```python
from build123d import *

# Parameters (mm, degrees)
F0_R     = 12.7
F1_DEPTH = 38.1
F3_DEPTH = 234.95
F5_DEPTH = 31.75
F6_SIZE  = 19.05


with BuildPart() as f1:
    # F0 (on Right) → F1 (new body)
    with BuildSketch(Plane.YZ):
        Polygon((0, 38.1), (0, 0), (50.8, 0), (50.8, 16.51), (31.75, 16.51), (31.75, 29.21), (50.8, 29.21), (50.8, 38.1), align=None)
        with BuildLine():
            Line((0, 50.8), (0, 38.1))
            Line((0, 38.1), (50.8, 38.1))
            Line((50.8, 38.1), (76.2, 38.1))
            Line((76.2, 38.1), (127, 38.1))
            Line((127, 38.1), (127, 50.8))
            Line((127, 50.8), (111.125, 50.8))
            Line((111.125, 50.8), (84.5934256055, 90.3501730104))
            ThreePointArc((84.5934256055, 90.3501730104), (63.5, 101.6), (42.4065743945, 90.3501730104))
            Line((42.4065743945, 90.3501730104), (15.875, 50.8))
            Line((15.875, 50.8), (0, 50.8))
        make_face()
        with Locations((63.5, 76.2)):
            Circle(F0_R, mode=Mode.SUBTRACT)
        Polygon((127, 38.1), (76.2, 38.1), (76.2, 29.21), (95.25, 29.21), (95.25, 16.51), (76.2, 16.51), (76.2, 0), (127, 0), align=None)
    extrude(amount=-F1_DEPTH)

    # F2 (on face) → F3 (join)
    with BuildSketch(Plane(origin=(-38.1, 0, 0), x_dir=(0, -1, 0), z_dir=(-1, 0, 0))):
        Polygon((0, 38.1), (-50.8, 38.1), (-50.8, 29.21), (-31.75, 29.21), (-31.75, 16.51), (-50.8, 16.51), (-50.8, 0), (0, 0), align=None)
        Polygon((-76.2, 38.1), (-127, 38.1), (-127, 0), (-76.2, 0), (-76.2, 16.51), (-95.25, 16.51), (-95.25, 29.21), (-76.2, 29.21), align=None)
    extrude(amount=F3_DEPTH)

    # F4 (on face) → F5 (join)
    with BuildSketch(Plane(origin=(-273.05, 0, 0), x_dir=(0, -1, 0), z_dir=(-1, 0, 0))):
        Polygon((-76.2, 16.51), (-76.2, 0), (0, 0), (0, 101.6), (-127, 101.6), (-127, 38.1), (-76.2, 38.1), (-76.2, 29.21), (-95.25, 29.21), (-95.25, 16.51), align=None)
        Polygon((-127, 38.1), (-127, 0), (-76.2, 0), (-76.2, 16.51), (-95.25, 16.51), (-95.25, 29.21), (-76.2, 29.21), (-76.2, 38.1), align=None)
    extrude(amount=F5_DEPTH)

    # F6
    f6_edges = [f1.edges().sort_by_distance(p)[0] for p in [
        (-304.8, 63.5, 101.6),
    ]]
    chamfer(f6_edges, length=F6_SIZE)


solid = f1.part
```
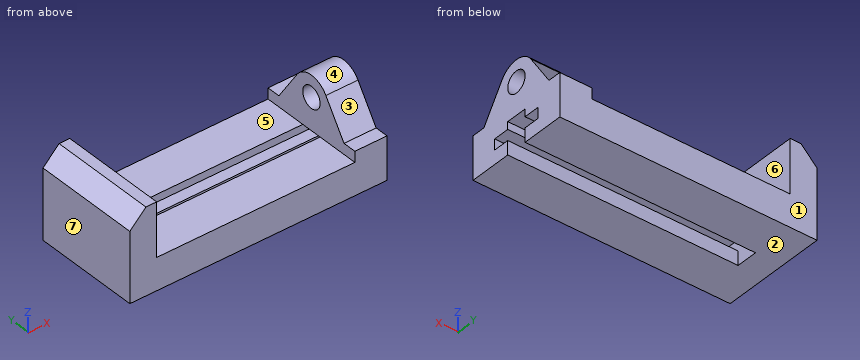
Check sheet for the modelled part. Datum: model origin and axes. Units: mm. Face numbers are marked on the shaded views. A direction names the side the tool comes from. Give positions to 0.01 mm unless a question says otherwise; leave off trailing zeros. Write each loop counter-clockwise with the first axis right and the second up, starting at its lowest first coordinate (ties: lowest second). Pieces come first, ordered by that corner, then holes. Notation, with made-up numbers: (5, -38) - (16, -38) arc R19 ccw to (16, -23) - close; hole circle Ø11 at (63.25, 28). An arc over 180 degrees is marked (long way). Answer as a JSON object with one key per item and string values. Group by question number.
1) Sectioned sample at C-C (z = 59). Record the cut outline in (x, y), then the cut area to 3 significant figures.
2) Thickness scan on probe 1 along Y at (x, z) = (-191, 6.5); probe 2 along X at (y, z) = (47.5, 80); probe 3 along Z at (x, y) = (-246.5, 94). Record the ranges inside material, lowest first. Write a range as from..to.
3) Sectioned sample at D-D (z = 76.2). Record the cut outline in (x, y), then the cut area to 3 significant figures.
4) Access from +Z, -Z, +X, -X, +Y, -Y to the whole of each face (thin tool, end or side, straight path). Record for the marked faces 4, 5, 6 and 7.
5) Sectioned sample at A-A (x = -147). Record the cut outline in (y, z).
6) Depth check by flat-ended pin: P1, Ø8, axis at x = -27, y = 117.5, coming from the +Z side. Enter the tip coordinate at first touch or a pass-through.
7) Sectioned sample at B-B (y = 63.5). Record the cut outline in (x, z).
8) Release check for a two-part mould opening along Z. For the marked faces 1, 2 and 3 record: pulls with the +Z half, pulls with the -Z half, needs draft (parallel to the pull), parting line crosses it, or undercut.
Geometry results:
{
 "1": {"outline": "(-304.8, 0) - (-273.05, 0) - (-273.05, 127) - (-304.8, 127) - close; (-38.1, 21.38) - (0, 21.38) - (0, 105.62) - (-38.1, 105.62) - close", "area": "7,240 mm^2"},
 "2": {"probe 1": "y = 0..50.8, 76.2..127", "probe 2": "x = -304.8..-273.05, -38.1..0", "probe 3": "z = 0..16.51, 29.21..38.1"},
 "3": {"outline": "(-304.8, 0) - (-273.05, 0) - (-273.05, 127) - (-304.8, 127) - close; (-38.1, 32.91) - (0, 32.91) - (0, 50.8) - (-38.1, 50.8) - close; (-38.1, 76.2) - (0, 76.2) - (0, 94.09) - (-38.1, 94.09) - close", "area": "5,400 mm^2"},
 "4": {"face 4": "+Z, +X", "face 5": "+Z, +Y, -Y", "face 6": "none", "face 7": "+Z, -Z, -X, +Y, -Y"},
 "5": {"outline": "(0, 0) - (50.8, 0) - (50.8, 16.51) - (31.75, 16.51) - (31.75, 29.21) - (50.8, 29.21) - (50.8, 38.1) - (0, 38.1) - close; (76.2, 0) - (127, 0) - (127, 38.1) - (76.2, 38.1) - (76.2, 29.21) - (95.25, 29.21) - (95.25, 16.51) - (76.2, 16.51) - close"},
 "6": {"P1": "stops at z = 50.8"},
 "7": {"outline": "(-304.8, 0) - (-273.05, 0) - (-273.05, 101.6) - (-285.75, 101.6) - (-304.8, 82.55) - close; (-38.1, 38.1) - (0, 38.1) - (0, 63.5) - (-38.1, 63.5) - close; (-38.1, 88.9) - (0, 88.9) - (0, 101.6) - (-38.1, 101.6) - close"},
 "8": {"face 1": "needs draft", "face 2": "pulls with the -Z half", "face 3": "pulls with the +Z half"}
}
